Autodesk Inventor part; units mm, degrees
ref_plane "YZ Plane" through (0, 0, 0) normal (1, 0, 0) x (0, 1, 0)
ref_plane "XZ Plane" through (0, 0, 0) normal (0, 1, 0) x (-1, 0, 0)
ref_plane "XY Plane" through (0, 0, 0) normal (0, 0, 1) x (1, 0, 0)
sketch "Sketch1" plane through (0, 0, 0) normal (0, 0, 1) x (1, 0, 0)
  line L0 (0, 0) -> (20, 0)
  line L1 (20, 0) -> (20, 14)
  line L2 (20, 14) -> (0, 14)
  line L3 (0, 14) -> (0, 0)
  dimension "d0" = 20
  dimension "d1" = 14
extrude "Extrusion1" add sketch "Sketch1" along normal blind 12
sketch "Sketch2" plane through (0, 0, 12) normal (0, 0, 1) x (1, 0, 0)
  line L0 (0, 0) -> (20, 0)
  line L1 (20, 14) -> (0, 14)
  line L2 (0, 14) -> (0, 0)
  line L3 (4.6094, 11.6352) -> (3.945, 9.5904)
  line L4 (3.945, 9.5904) -> (1.795, 9.5904)
  line L5 (1.795, 9.5904) -> (1.1306, 11.6352)
  line L6 (1.1306, 11.6352) -> (2.87, 12.8989)
  line L7 (2.87, 12.8989) -> (4.6094, 11.6352)
  line L8 (18.8694, 11.6352) -> (18.205, 9.5904)
  line L9 (18.205, 9.5904) -> (16.055, 9.5904)
  line L10 (16.055, 9.5904) -> (15.3906, 11.6352)
  line L11 (15.3906, 11.6352) -> (17.13, 12.8989)
  line L12 (17.13, 12.8989) -> (18.8694, 11.6352)
  line L13 (4.6094, 3.4952) -> (3.945, 1.4504)
  line L14 (3.945, 1.4504) -> (1.795, 1.4504)
  line L15 (1.795, 1.4504) -> (1.1306, 3.4952)
  line L16 (1.1306, 3.4952) -> (2.87, 4.7589)
  line L17 (2.87, 4.7589) -> (4.6094, 3.4952)
  line L18 (18.8694, 3.4952) -> (18.205, 1.4504)
  line L19 (18.205, 1.4504) -> (16.055, 1.4504)
  line L20 (16.055, 1.4504) -> (15.3906, 3.4952)
  line L21 (15.3906, 3.4952) -> (17.13, 4.7589)
  line L22 (17.13, 4.7589) -> (18.8694, 3.4952)
  point P0 (2.87, 11.07)
  point P1 (17.13, 11.07)
  point P2 (2.87, 2.93)
  point P3 (17.13, 2.93)
  dimension "d14" = 2.15
  dimension "d16" = 2.15
  dimension "d17" = 2.93
  dimension "d18" = 2.87
  dimension "d20" = 2.93
  dimension "d55" = 2.15
  dimension "d56" = 2.15
extrude "Extrusion2" add sketch "Sketch2" along normal blind 4
chamfer "Chamfer1" distance 0.5 angle 45 20 edges at (4.2772, 10.6128, 16) (2.87, 9.5904, 16) (1.4628, 10.6128, 16) (2.0003, 12.267, 16) (3.7397, 12.267, 16) (3.7397, 4.127, 16) (2.0003, 4.127, 16) (1.4628, 2.4728, 16) (2.87, 1.4504, 16) (4.2772, 2.4728, 16) (17.13, 1.4504, 16) (15.7228, 2.4728, 16) (16.2603, 4.127, 16) (17.9997, 4.127, 16) (18.5372, 2.4728, 16) (17.13, 9.5904, 16) (18.5372, 10.6128, 16) (17.9997, 12.267, 16) (16.2603, 12.267, 16) (15.7228, 10.6128, 16)
sketch "Sketch3" plane through (0, 0, 0) normal (0, 0, -1) x (-1, 0, 0)
  line L0 (0, 0) -> (-20, 0)
  line L1 (0, 14) -> (0, 0)
  line L2 (-20, 14) -> (0, 14)
  line L3 (-20, 0) -> (-20, 14)
  line L4 (-4.8116, 3.5609) -> (-2.87, 4.9716)
  line L5 (-2.87, 4.9716) -> (-0.9284, 3.5609)
  line L6 (-0.9284, 3.5609) -> (-1.67, 1.2783)
  line L7 (-1.67, 1.2783) -> (-4.07, 1.2783)
  line L8 (-4.07, 1.2783) -> (-4.8116, 3.5609)
  line L9 (-19.0716, 3.5609) -> (-17.13, 4.9716)
  line L10 (-17.13, 4.9716) -> (-15.1884, 3.5609)
  line L11 (-15.1884, 3.5609) -> (-15.93, 1.2783)
  line L12 (-15.93, 1.2783) -> (-18.33, 1.2783)
  line L13 (-18.33, 1.2783) -> (-19.0716, 3.5609)
  line L14 (-2.87, 13.1116) -> (-0.9284, 11.7009)
  line L15 (-0.9284, 11.7009) -> (-1.67, 9.4183)
  line L16 (-1.67, 9.4183) -> (-4.07, 9.4183)
  line L17 (-4.07, 9.4183) -> (-4.8116, 11.7009)
  line L18 (-4.8116, 11.7009) -> (-2.87, 13.1116)
  line L19 (-17.13, 13.1116) -> (-15.1884, 11.7009)
  line L20 (-15.1884, 11.7009) -> (-15.93, 9.4183)
  line L21 (-15.93, 9.4183) -> (-18.33, 9.4183)
  line L22 (-18.33, 9.4183) -> (-19.0716, 11.7009)
  line L23 (-19.0716, 11.7009) -> (-17.13, 13.1116)
  point P0 (-2.87, 2.93)
  point P1 (-17.13, 2.93)
  point P2 (-2.87, 11.07)
  point P3 (-17.13, 11.07)
  dimension "d30" = 2.4
  dimension "d31" = 2.4
  dimension "d32" = 2.4
  dimension "d33" = 2.4
  dimension "d34" = 2.87
  dimension "d35" = 2.87
  dimension "d36" = 2.93
  dimension "d37" = 2.93
extrude "Extrusion3" cut sketch "Sketch3" against normal blind 4.5 contours L4 L5 L6 L7 L8 | L9 L10 L11 L12 L13 | L14 L15 L16 L17 L18 | L19 L20 L21 L22 L23
chamfer "Chamfer2" distance 0.5 angle 45 20 edges at (17.13, 1.2783, 0) (18.7008, 2.4196, 0) (15.5592, 2.4196, 0) (16.1592, 4.2662, 0) (18.1008, 4.2662, 0) (1.8992, 4.2662, 0) (1.2992, 2.4196, 0) (2.87, 1.2783, 0) (4.4408, 2.4196, 0) (3.8408, 4.2662, 0) (4.4408, 10.5596, 0) (2.87, 9.4183, 0) (1.2992, 10.5596, 0) (1.8992, 12.4062, 0) (3.8408, 12.4062, 0) (16.1592, 12.4062, 0) (15.5592, 10.5596, 0) (17.13, 9.4183, 0) (18.7008, 10.5596, 0) (18.1008, 12.4062, 0)
sketch "Sketch5" plane through (0, 0, 12) normal (0, 0, 1) x (1, 0, 0)
  line L0 (20, 14) -> (0, 14)
  line L1 (0, 14) -> (0, 0)
  line L2 (4.5, 8.3) -> (15.5, 8.3)
  line L3 (15.5, 8.3) -> (15.5, 5.7)
  line L4 (15.5, 5.7) -> (4.5, 5.7)
  line L5 (4.5, 5.7) -> (4.5, 8.3)
  dimension "d60" = 11
  dimension "d61" = 2.6
  dimension "d62" = 5.7
  dimension "d63" = 4.5
extrude "Extrusion5" cut sketch "Sketch5" against normal up to next
properties part number "lego"
Check sheet for the modelled part. Datum: model origin and axes. Units: mm. A direction names the side the tool comes from. Round coordinates to 2 decimals unless told otherwise and drop trailing zeros. Order: outer loops, then holes, each group sorted by start corner. A loop starts at its lowest first (then second) coordinate and runs counter-clockwise, first axis right, second up.
1) Section check B-B (x = 7). Record the boundary of the cut face in (y, z), and give its area (3 significant figures).
2) Section check A-A (z = 7). Record the boundary of the cut face in (x, y).
3) Mould release check, pull along Y, two halves, no side actions. Record for faces 1 (the flat face through (10, 8.3, 6)), 2 (the flat face through (17, 3, 16)), 3 (the flat face through (3.603, 12.053, 15.753)): +Y half, -Y half, draft (parallel to the pull), parting line (faces both ways), or undercut.
4) Go/stop test with flat-tipped pins: pin 1 Ø6 at (x, z) = (8, 11) entering from -Y; pin 2 Ø1.1 at (x, z) = (16.5, 13.5) entering from -Y; pin 3 Ø4 at (x, y) = (9, 5) entering from +Z. Record where each tip stops, or that it passes through.
5) Tool access check on faces 4 (the flat face through (16.25, 4.12, 13.73)), 5 (the flat face through (17, 9.59, 14)), 6 (the flat face through (3, 1.278, 2)). Record the directions out of +Z, -Z, +X, -X, +Y, -Y that give a thin tool (end or side, any length) a straight path to the whole face; none if there is none.
6) Section check C-C (y = 6.25). Record the boundary of the cut face in (x, z).
7) Section check D-D (z = 13.75). Record the boundary of the cut face in (x, y) (3 decimals).
8) Scan lines: line 1 (Y direction, x = 5, z = 5); line 2 (X direction, y = 5.75, z = 10.25); line 3 (Y direction, x = 3.5, z = 2). Record each from-to range of solid material in increasing order.
Result:
1. outline: (0, 0) - (5.7, 0) - (5.7, 12) - (0, 12) - close; (8.3, 0) - (14, 0) - (14, 12) - (8.3, 12) - close
1. area: 137 mm2
2. outline: (0, 0) - (20, 0) - (20, 14) - (0, 14) - close; hole (4.5, 5.7) - (15.5, 5.7) - (15.5, 8.3) - (4.5, 8.3) - close
3. face 1: undercut
3. face 2: draft
3. face 3: +Y half
4. pin 1: stops at y = 0
4. pin 2: stops at y = 1.45
4. pin 3: stops at z = 12
5. face 4: +Z
5. face 5: +Z, +X, -X
5. face 6: -Z
6. outline: (0, 0) - (4.5, 0) - (4.5, 12) - (0, 12) - close; (15.5, 0) - (20, 0) - (20, 12) - (15.5, 12) - close
7. outline: (1.131, 3.495) - (1.795, 1.45) - (3.945, 1.45) - (4.609, 3.495) - (2.87, 4.759) - close; (1.131, 11.635) - (1.795, 9.59) - (3.945, 9.59) - (4.609, 11.635) - (2.87, 12.899) - close; (15.391, 3.495) - (16.055, 1.45) - (18.205, 1.45) - (18.869, 3.495) - (17.13, 4.759) - close; (15.391, 11.635) - (16.055, 9.59) - (18.205, 9.59) - (18.869, 11.635) - (17.13, 12.899) - close
8. line 1: y = 0 to 5.7, 8.3 to 14
8. line 2: x = 0 to 4.5, 15.5 to 20
8. line 3: y = 0 to 1.28, 4.51 to 9.42, 12.65 to 14
